from build123d import *

# Parameters (mm, degrees)
F0_W     = 350
F0_H     = 140
F1_DEPTH = 20
F2_R     = 12.5
F3_DEPTH = 5
F4_R     = 2
F5_R     = 5
F6_R     = 2


with BuildPart() as f1:
    # F0 (on Top) → F1 (new body)
    with BuildSketch(Plane.XY):
        Rectangle(F0_W, F0_H)
    extrude(amount=F1_DEPTH)

    # F2 (on face) → F3 (join)
    with BuildSketch(Plane(origin=(0, 0, 0), x_dir=(1, 0, 0), z_dir=(0, 0, -1))):
        with Locations((145, 40)):
            Circle(F2_R)
        with Locations((145, -40)):
            Circle(F2_R)
        with Locations((-145, 40)):
            Circle(F2_R)
        with Locations((-145, -40)):
            Circle(F2_R)
    extrude(amount=F3_DEPTH)

    # F4
    f4_edges = [f1.edges().sort_by_distance(p)[0] for p in [
        (-157.5, -40, -5),
        (-157.5, 40, -5),
        (132.5, 40, -5),
        (132.5, -40, -5),
    ]]
    fillet(f4_edges, radius=F4_R)

    # F5
    f5_edges = [f1.edges().sort_by_distance(p)[0] for p in [
        (-175, -70, 10),
        (-175, 70, 10),
        (175, -70, 10),
        (175, 70, 10),
    ]]
    fillet(f5_edges, radius=F5_R)

    # F6
    f6_edges = [f1.edges().sort_by_distance(p)[0] for p in [
        (175, 0, 20),
    ]]
    fillet(f6_edges, radius=F6_R)


solid = f1.part
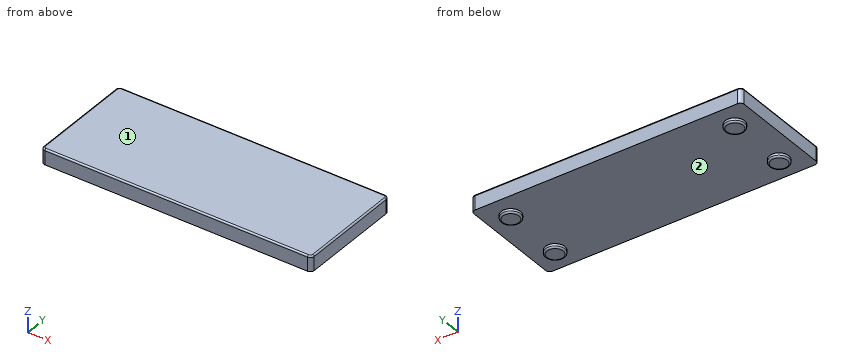
Geometry check sheet. Reference: the model listing, model coordinates, mm. Face numbers are marked on the shaded views. Round coordinates to 2 decimals unless told otherwise and drop trailing zeros. Loops run counter-clockwise (first coordinate to the right, second up) from the corner with the lowest first, then second, coordinate; pieces in that order, holes last.
Item 1: Mould release check, pull along X, two halves, no side actions. Record for the marked faces 1 and 2: pulls with the +X half, pulls with the -X half, needs draft (parallel to the pull), parting line crosses it, or undercut.
Item 2: Thickness scan on line 1 (Z direction, x = -126, y = 16.5); line 2 (Y direction, x = 158.5, z = 19); line 3 (X direction, y = -30, z = -2.5). Record the ranges inside material, lowest first.
Item 3: Cross-section at C-C on y = 40. Record the boundary of the cut face in (x, z).
Item 4: Cross-section at D-D on x = -59. Record the boundary of the cut face in (y, z).
Item 5: Cross-section at B-B on x = 145. Record the boundary of the cut face in (y, z).
Item 6: Cross-section at A-A on y = -10. Record the boundary of the cut face in (x, z).
Item 7: Gauge pin test, flat end, axial feed: pin 1 (1 mm diameter, centred on x = -101.5, y = -30, fed in from -Z). Record the tip position at first contact, or that the pin passes through.
Answer sheet:
1. face 1: needs draft
1. face 2: undercut
2. line 1: z = 0 to 20
2. line 2: y = -69.73 to 69.73
2. line 3: x = -152.5 to -137.5, 137.5 to 152.5
3. outline: (-175, 0) - (-157.5, 0) - (-157.5, -3) arc R2 ccw to (-155.5, -5) - (-134.5, -5) arc R2 ccw to (-132.5, -3) - (-132.5, 0) - (132.5, 0) - (132.5, -3) arc R2 ccw to (134.5, -5) - (155.5, -5) arc R2 ccw to (157.5, -3) - (157.5, 0) - (175, 0) - (175, 18) arc R2 ccw to (173, 20) - (-173, 20) arc R2 ccw to (-175, 18) - close
4. outline: (-70, 0) - (70, 0) - (70, 18) arc R2 ccw to (68, 20) - (-68, 20) arc R2 ccw to (-70, 18) - close
5. outline: (-70, 0) - (-52.5, 0) - (-52.5, -3) arc R2 ccw to (-50.5, -5) - (-29.5, -5) arc R2 ccw to (-27.5, -3) - (-27.5, 0) - (27.5, 0) - (27.5, -3) arc R2 ccw to (29.5, -5) - (50.5, -5) arc R2 ccw to (52.5, -3) - (52.5, 0) - (70, 0) - (70, 18) arc R2 ccw to (68, 20) - (-68, 20) arc R2 ccw to (-70, 18) - close
6. outline: (-175, 0) - (175, 0) - (175, 18) arc R2 ccw to (173, 20) - (-173, 20) arc R2 ccw to (-175, 18) - close
7. pin 1: stops at z = 0
